Read the model definition and answer for the solid it produces. Units are mm, in the model's axes. A direction names the side the tool comes from. Give positions to 0.01 mm unless a question says otherwise; leave off trailing zeros. Order: outer loops, then holes, each group sorted by start corner. A loop starts at its lowest first (then second) coordinate and runs counter-clockwise, first axis right, second up. Notation, with made-up numbers: (25, -22.75) - (74, -22.75) arc R15 ccw to (74, -13.75) - close; hole circle Ø11 at (-35.5, -28). An arc over 180 degrees is marked (long way). Write item = value, one per line.
Autodesk Inventor part; units mm, degrees
ref_plane "YZ Plane" through (0, 0, 0) normal (1, 0, 0) x (0, 1, 0)
ref_plane "XZ Plane" through (0, 0, 0) normal (0, 1, 0) x (-1, 0, 0)
ref_plane "XY Plane" through (0, 0, 0) normal (0, 0, 1) x (1, 0, 0)
sketch "Sketch1" plane through (0, 0, 0) normal (0, 1, 0) x (-1, 0, 0)
  arc A0 (10.9086, 1.7618) -> (10.9086, -1.7618) centre (0, 0) ccw
  arc A1 (14.3065, 2.361) -> (14.3065, -2.361) centre (0, 0) ccw
  line L0 (15, 13.2439) -> (15, 20)
  line L1 (15, 20) -> (18, 20)
  line L2 (18, 20) -> (18, 8)
  line L3 (15, -13.2439) -> (15, -20)
  line L4 (15, -20) -> (18, -20)
  line L5 (18, -20) -> (18, -8)
  arc A2 (9.6355, 10.8355) -> (15, 13.2439) centre (11.7771, 13.2439) ccw
  arc A3 (15, -13.2439) -> (9.6355, -10.8355) centre (11.7771, -13.2439) ccw
  line L6 (10.9086, -1.7618) -> (14.3065, -2.361)
  line L7 (10.9086, 1.7618) -> (14.3065, 2.361)
  line L8 (17.4762, 0) -> (-4.0395, 0) construction
  arc A4 (18, 8) -> (14.3065, 2.361) centre (19.2199, 3.1718) ccw
  arc A5 (14.3065, -2.361) -> (18, -8) centre (19.2199, -3.1718) ccw
  dimension "d0" = 22.1
  dimension "d1" = 29
  dimension "d2" = 12
  dimension "d3" = 12
  dimension "d4" = 3
  dimension "d5" = 3
  dimension "d8" = 15
  dimension "d10" = 10
  dimension "d11" = 10
  dimension "d12" = 3.5237
  dimension "d13" = 1.7618
  dimension "d14" = 20
  dimension "d15" = 20
extrude "Extrusion1" add sketch "Sketch1" along normal blind 30
equation "\"d3\" = d2"
equation "\"d11\" = d10"
equation "\"d13\" = 0.5 * d12"
properties part number "motor_holder" material "ABS Plastic"
1. For faces 5 (the face through (-12.584, 14.79, -2.057)), 6 (the face through (-15, 15, -17)), 7 (the face through (-16, 15, -20)), determine the directions among +Z, -Z, +X, -X, +Y, -Y from which every point of the face is accessible in a straight line to the end or side of a thin tool.
Recorded:
face_5 = -X, +Y, -Y
face_6 = -Z, +Y, -Y
face_7 = -Z, +X, -X, +Y, -Y
2. Section C-C (x = -8.5) is taken. Determine the outline of the cut face in (y, z).
Recorded:
outline = (0, -11.75) - (30, -11.75) - (30, -7.06) - (0, -7.06) - close; (0, 7.06) - (30, 7.06) - (30, 11.75) - (0, 11.75) - close
3. Flat-ended cylindrical pins translate along their axes: pin 1 (2 mm diameter, centred on x = -1, y = 19.5, fed in from +Z); pin 2 (7.5 mm diameter, centred on y = 20.5, z = 15.5, fed in from +X); pin 3 (6 mm diameter, centred on x = 4.5, y = 23.5, fed in from -Z). Find the tip coordinate at first contact, or state that the pin passes through.
Recorded:
pin_1 = 14.5
pin_2 = 8.5
pin_3 = -14.42
4. Determine the mould class of faces 1 (the face through (-18, 15, -14)), 2 (the face through (-11, 30, 3)), 3 (the face through (-15, 15, 17)), 4 (the face through (-13.05, 14.79, -10.283)) for opening direction X: +X half, -X half, draft (parallel to the pull), parting line (faces both ways), or undercut.
Recorded:
face_1 = -X half
face_2 = draft
face_3 = undercut
face_4 = undercut
5. Section A-A (x = 0) is taken. Determine the outline of the cut face in (y, z), and give its area (3 significant figures).
Recorded:
outline = (0, -14.5) - (30, -14.5) - (30, -11.05) - (0, -11.05) - close; (0, 11.05) - (30, 11.05) - (30, 14.5) - (0, 14.5) - close
area = 207 mm^2
6. Section B-B (y = 6.75) is taken. Determine the outline of the cut face in (x, z), and give its area (3 significant figures).
Recorded:
outline = (-18, -20) - (-15, -20) - (-15, -13.24) arc R3.22 cw to (-9.64, -10.84) arc R14.5 ccw (long way) to (-9.64, 10.84) arc R3.22 cw to (-15, 13.24) - (-15, 20) - (-18, 20) - (-18, 8) arc R4.98 cw to (-14.31, 2.36) - (-10.91, 1.76) arc R11.05 cw (long way) to (-10.91, -1.76) - (-14.31, -2.36) arc R4.98 cw to (-18, -8) - close
area = 373 mm^2
7. Straight lines are drawn through the part: L1, parallel to Z at x = 0, y = 17.5; L2, parallel to Z at x = 3.5, y = 19.75; L3, parallel to X at y = 14.25, z = 17.5. For each, find the intervals that lie inside material, in ascending order. Write a range as [from, to].
Recorded:
L1 = [-14.5, -11.05], [11.05, 14.5]
L2 = [-14.07, -10.48], [10.48, 14.07]
L3 = [-18, -15]
8. Section D-D (z = 0) is taken. Determine the outline of the cut face in (x, y), and give its area (3 significant figures).
Recorded:
outline = (11.05, 0) - (14.5, 0) - (14.5, 30) - (11.05, 30) - close
area = 104 mm^2
